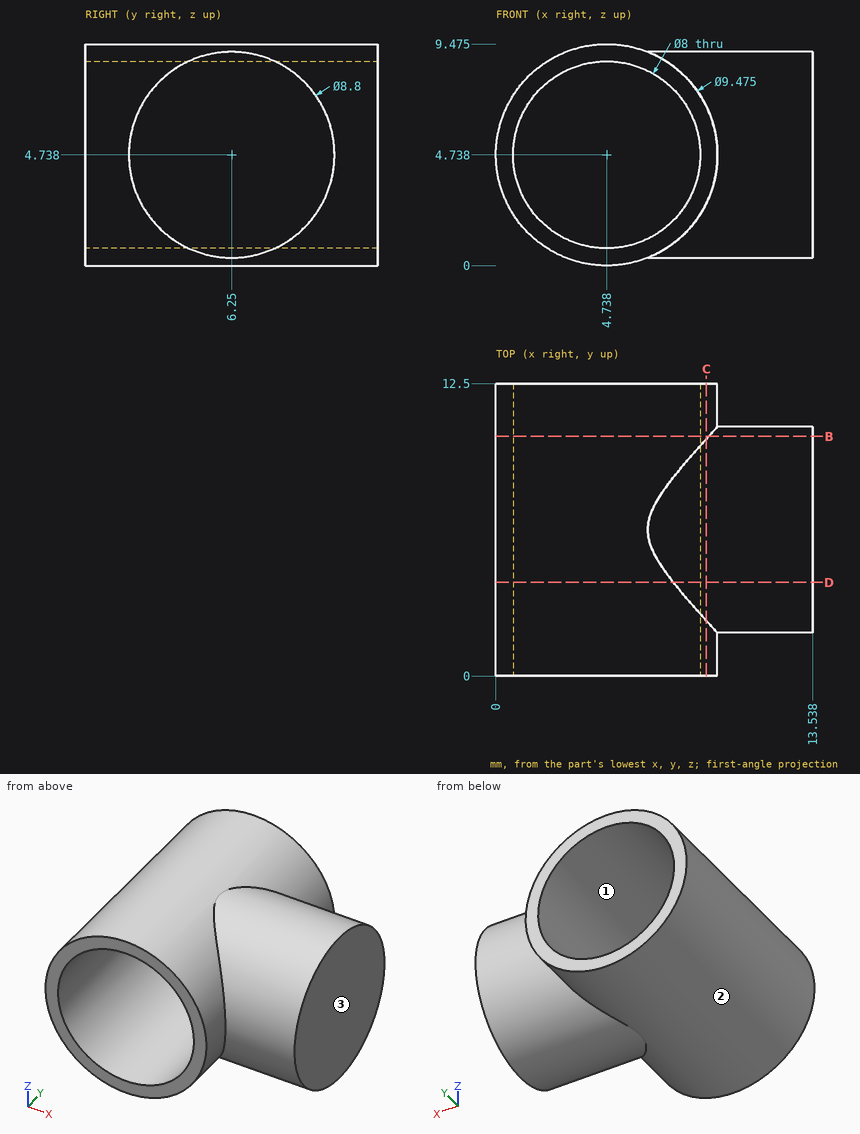
Input: dimensioned drawing with shaded views. Units: mm. Origin: part minimum x, y, z. Round coordinates to 2 decimals unless told otherwise and drop trailing zeros. Order: outer loops, then holes, each group sorted by start corner. A loop starts at its lowest first (then second) coordinate and runs counter-clockwise, first axis right, second up.
1. Cut plane C-C, the plane x = 9. Output: boundary loops of the cut face in (y, z).
The answers:
outline: (0, 2.67) - (2.37, 2.67) arc R4.4 ccw to (10.13, 2.67) - (12.5, 2.67) - (12.5, 6.81) - (10.13, 6.81) arc R4.4 ccw to (2.37, 6.81) - (0, 6.81) - close
2. Material intervals for line 1 (X direction, y = 5, z = 4.75); line 2 (Z direction, x = 3.75, y = 2) (1 decimal); line 3 (Z direction, x = 2, y = 1) (1 decimal), sorted ascending.
The answers:
line 1: x = 0 to 0.74, 8.74 to 13.54
line 2: z = 0.1 to 0.9, 8.6 to 9.4
line 3: z = 0.9 to 1.8, 7.7 to 8.6
3. Mould query, pull axis Z, two halves, no side actions, for the marked faces 1, 2 and 3. Classes: released by +Z, released by -Z, zero draft, split by the parting line, or undercut.
The answers:
face 1: undercut
face 2: split by the parting line
face 3: zero draft
4. Pin query (flat end, axial travel): P1, Ø3, axis at y = 4.5, z = 5, coming from the -X side. Return the tip coordinate at first contact, or that it passes through.
The answers:
P1: stops at x = 0
5. Cut plane D-D, the plane y = 4. Output: boundary loops of the cut face in (x, z) (1 decimal).
The answers:
outline: (7.6, 1) - (13.5, 1) - (13.5, 8.5) - (7.6, 8.5) arc R4.7 ccw (long way) to start; hole circle Ø8 at (4.7, 4.7)
6. Cut plane B-B, the plane y = 10.25. Output: boundary loops of the cut face in (x, z) (1 decimal).
The answers:
outline: (9.1, 2.9) - (13.5, 2.9) - (13.5, 6.6) - (9.1, 6.6) arc R4.7 ccw (long way) to start; hole circle Ø8 at (4.7, 4.7)
